```python
from build123d import *

# Parameters (mm, degrees)
BOSS_EXTRUDE1_DEPTH = 2


with BuildPart() as part:
    # Sketch1 → Boss-Extrude1 (new body)
    with BuildSketch(Plane(origin=(0, 0, 0), x_dir=(1, 0, 0), z_dir=(0, 1, 0))):
        with BuildLine():
            ThreePointArc((-5.123475383, 4), (-6.146242348, 2.115113473), (-6.5, 0))
            Line((-6.5, 0), (-1.75, 0))
            ThreePointArc((-1.75, 0), (-1.237436867, 1.237436867), (0, 1.75))
            Line((0, 1.75), (0, 4))
            Line((0, 4), (-5.123475383, 4))
        make_face()
        with BuildLine():
            Line((0, 4), (0, 1.75))
            ThreePointArc((0, 1.75), (1.237436867, 1.237436867), (1.75, 0))
            Line((1.75, 0), (6.5, 0))
            ThreePointArc((6.5, 0), (6.146242348, 2.115113473), (5.123475383, 4))
            Line((5.123475383, 4), (0, 4))
        make_face()
        with BuildLine():
            Line((-1.75, 0), (-6.5, 0))
            ThreePointArc((-6.5, 0), (-6.146242348, -2.115113473), (-5.123475383, -4))
            Line((-5.123475383, -4), (0, -4))
            Line((0, -4), (0, -1.75))
            ThreePointArc((0, -1.75), (-1.237436867, -1.237436867), (-1.75, 0))
        make_face()
        with BuildLine():
            Line((0, -1.75), (0, -4))
            Line((0, -4), (5.123475383, -4))
            ThreePointArc((5.123475383, -4), (6.146242348, -2.115113473), (6.5, 0))
            Line((6.5, 0), (1.75, 0))
            ThreePointArc((1.75, 0), (1.237436867, -1.237436867), (0, -1.75))
        make_face()
    extrude(amount=BOSS_EXTRUDE1_DEPTH)


solid = part.part
```
Model file for the job. Use its own axes, mm. Coordinates: 2 decimals unless noted, no trailing zeros. Order: outer loops, then holes, each group sorted by start corner. A loop starts at its lowest first (then second) coordinate and runs counter-clockwise, first axis right, second up. Notation, with made-up numbers: M 41,-6 L 98,-6 A11 cw 98,9 Z; hole C 73,76.25 d2. An arc over 180 degrees is marked long. Answer as CSV lines item,"result".
(1) Band-saw the part on C-C, the plane z = 0.5. List the corners of the cut face in (x, y), then the cut area to 3 significant figures.
Geometry says:
outline,"M -6.48,0 L -1.68,0 L -1.68,2 L -6.48,2 Z; M 1.68,0 L 6.48,0 L 6.48,2 L 1.68,2 Z"
area,"19.2 mm2"
(2) Band-saw the part on A-A, the plane y = 1.15. List the corners of the cut face in (x, z).
Geometry says:
outline,"M -5.12,-4 L 5.12,-4 A6.5 ccw 5.12,4 L -5.12,4 A6.5 ccw Z; hole C 0,0 d3.5"
(3) Band-saw the part on D-D, the plane x = -5.25. List the corners of the cut face in (y, z), then the cut area to 3 significant figures.
Geometry says:
outline,"M 0,-3.83 L 2,-3.83 L 2,3.83 L 0,3.83 Z"
area,"15.3 mm2"
(4) Wall check: line 1 along Z through (x, y) = (-0.5, 0.8); line 2 along X through (y, z) = (1.3, 1); line 3 along X through (y, z) = (1.25, -0.5). Give the ranges that are in metal, low to high.
Geometry says:
line 1,"z = -4 to -1.68, 1.68 to 4"
line 2,"x = -6.42 to -1.44, 1.44 to 6.42"
line 3,"x = -6.48 to -1.68, 1.68 to 6.48"
(5) Band-saw the part on B-B, the plane x = 0.75. List the corners of the cut face in (y, z).
Geometry says:
outline,"M 0,-4 L 2,-4 L 2,-1.58 L 0,-1.58 Z; M 0,1.58 L 2,1.58 L 2,4 L 0,4 Z"
